```python
from build123d import *

# Parameters (mm, degrees)
SKETCH_1_R      = 2.05
EXTRUDE_1_DEPTH = 3
FILLET_1_R      = 1


with BuildPart() as part:
    # 草图1 → 凸台-拉伸1 (new body)
    with BuildSketch(Plane.XY):
        with BuildLine():
            Line((8, -14.5), (11.5, -14.5))
            Line((11.5, -14.5), (11.5, -12.41))
            ThreePointArc((11.5, -12.41), (10.495, -11.405), (11.5, -10.4))
            Line((11.5, -10.4), (14.5, -10.4))
            Line((14.5, -10.4), (14.5, -3.6))
            Line((14.5, -3.6), (11.5, -3.6))
            ThreePointArc((11.5, -3.6), (10.495, -2.595), (11.5, -1.59))
            Line((11.5, -1.59), (11.5, 1.59))
            ThreePointArc((11.5, 1.59), (10.495, 2.595), (11.5, 3.6))
            Line((11.5, 3.6), (14.5, 3.6))
            Line((14.5, 3.6), (14.5, 10.4))
            Line((14.5, 10.4), (11.5, 10.4))
            ThreePointArc((11.5, 10.4), (10.495, 11.405), (11.5, 12.41))
            Line((11.5, 12.41), (11.5, 14.5))
            Line((11.5, 14.5), (7, 14.5))
            ThreePointArc((7, 14.5), (5.95, 13.45), (4.9, 14.5))
            Line((4.9, 14.5), (4.9, 17.5))
            Line((4.9, 17.5), (-4.9, 17.5))
            Line((-4.9, 17.5), (-4.9, 14.5))
            ThreePointArc((-4.9, 14.5), (-5.95, 13.45), (-7, 14.5))
            Line((-7, 14.5), (-11.5, 14.5))
            Line((-11.5, 14.5), (-11.5, 12.41))
            ThreePointArc((-11.5, 12.41), (-10.789357685, 12.115642315), (-10.495, 11.405))
            ThreePointArc((-10.495, 11.405), (-10.789357685, 10.694357685), (-11.5, 10.4))
            Line((-11.5, 10.4), (-14.5, 10.4))
            Line((-14.5, 10.4), (-14.5, 3.6))
            Line((-14.5, 3.6), (-11.5, 3.6))
            ThreePointArc((-11.5, 3.6), (-10.789357685, 3.305642315), (-10.495, 2.595))
            ThreePointArc((-10.495, 2.595), (-10.789357685, 1.884357685), (-11.5, 1.59))
            Line((-11.5, 1.59), (-11.5, -1.59))
            ThreePointArc((-11.5, -1.59), (-10.789357685, -1.884357685), (-10.495, -2.595))
            ThreePointArc((-10.495, -2.595), (-10.789357685, -3.305642315), (-11.5, -3.6))
            Line((-11.5, -3.6), (-14.5, -3.6))
            Line((-14.5, -3.6), (-14.5, -10.4))
            Line((-14.5, -10.4), (-11.5, -10.4))
            ThreePointArc((-11.5, -10.4), (-10.789357685, -10.694357685), (-10.495, -11.405))
            ThreePointArc((-10.495, -11.405), (-10.789357685, -12.115642315), (-11.5, -12.41))
            Line((-11.5, -12.41), (-11.5, -14.5))
            Line((-11.5, -14.5), (-8, -14.5))
            ThreePointArc((-8, -14.5), (-6.95, -13.45), (-5.9, -14.5))
            Line((-5.9, -14.5), (-5.9, -17.5))
            Line((-5.9, -17.5), (5.9, -17.5))
            Line((5.9, -17.5), (5.9, -14.5))
            ThreePointArc((5.9, -14.5), (6.95, -13.45), (8, -14.5))
        make_face()
        with Locations((-7, -7)):
            Circle(SKETCH_1_R, mode=Mode.SUBTRACT)
        with Locations((7, -7)):
            Circle(SKETCH_1_R, mode=Mode.SUBTRACT)
        Polygon((-7.5, 0.890105817), (-7.5, 8.609894183), (-2.465355414, 4.75), align=None, mode=Mode.SUBTRACT)
        Polygon((5.034644586, -1), (-5.034644586, -1), (0, 2.859894183), align=None, mode=Mode.SUBTRACT)
        Polygon((-5.034644586, 10.5), (5.034644586, 10.5), (0, 6.640105817), align=None, mode=Mode.SUBTRACT)
        Polygon((2.465355414, 4.75), (7.5, 8.609894183), (7.5, 0.890105817), align=None, mode=Mode.SUBTRACT)
    extrude(amount=EXTRUDE_1_DEPTH)

    # 圆角1
    fillet_1_edges = [part.edges().sort_by_distance(p)[0] for p in [
        (5.034644586, -1, 1.5),
        (0, 2.859894183, 1.5),
        (-7.5, 8.609894183, 1.5),
        (-7.5, 0.890105817, 1.5),
        (-2.465355414, 4.75, 1.5),
        (0, 6.640105817, 1.5),
        (5.034644586, 10.5, 1.5),
        (-5.034644586, 10.5, 1.5),
        (7.5, 0.890105817, 1.5),
        (7.5, 8.609894183, 1.5),
        (2.465355414, 4.75, 1.5),
        (-5.034644586, -1, 1.5),
    ]]
    fillet(fillet_1_edges, radius=FILLET_1_R)


solid = part.part
```
Design review of the part built by this model. Coordinates are the model's own, in mm. A direction names the side the tool comes from. Give positions to 0.01 mm unless a question says otherwise; leave off trailing zeros. Write each loop counter-clockwise with the first axis right and the second up, starting at its lowest first coordinate (ties: lowest second). Pieces come first, ordered by that corner, then holes.
(1) Add section B-B (y = -5.5). Give the boundary of the cut face in (x, z), and give its area (3 significant figures).
Checked values:
outline: (-14.5, 0) - (-8.4, 0) - (-8.4, 3) - (-14.5, 3) - close; (-5.6, 0) - (5.6, 0) - (5.6, 3) - (-5.6, 3) - close; (8.4, 0) - (14.5, 0) - (14.5, 3) - (8.4, 3) - close
area: 70.2 mm2
(2) Add section A-A (x = 0). Give the boundary of the cut face in (y, z), and give its area (3 significant figures).
Checked values:
outline: (-17.5, 0) - (-1, 0) - (-1, 3) - (-17.5, 3) - close; (2.6, 0) - (6.9, 0) - (6.9, 3) - (2.6, 3) - close; (10.5, 0) - (17.5, 0) - (17.5, 3) - (10.5, 3) - close
area: 83.4 mm2
(3) Add section D-D (y = -2). Give the boundary of the cut face in (x, z), and give its area (3 significant figures).
Checked values:
outline: (-10.69, 0) - (10.69, 0) - (10.69, 3) - (-10.69, 3) - close
area: 64.1 mm2
(4) Wall thickness on line 1 along Y through (x, z) = (-2, 2.35); line 2 along Y through (x, z) = (0.5, 0.65); line 3 along X through (y, z) = (14, 2): over which ranges is each line inside the solid? List them lowest first.
Checked values:
line 1: y = -17.5 to -1, 1.33 to 8.17, 10.5 to 17.5
line 2: y = -17.5 to -1, 2.47 to 7.03, 10.5 to 17.5
line 3: x = -11.5 to -6.87, -5.03 to 5.03, 6.87 to 11.5
(5) Mouldability with a two-part tool opening along Y and no side actions: class faces 4 (the face through (6.93, -13.45, 1.48)), 5 (the face through (-11.5, 13, 1)), 6 (the face through (-1.67, 1.58, 1.48)) as +Y half, -Y half, draft (parallel to the pull), parting line (faces both ways), or undercut.
Checked values:
face 4: -Y half
face 5: draft
face 6: undercut
(6) Clearance check with flat-ended pins moving along their axes: pin 1 Ø0.9 at (x, z) = (13, 1) entering from +Y; pin 2 Ø1.7 at (y, z) = (-13, 1) entering from +X; pin 3 Ø1 at (x, y) = (6.5, -3.5) entering from -Z; pin 4 Ø0.9 at (x, z) = (-13, 1.5) entering from -Y. State where each tip first meets the part, or that it passes through.
Checked values:
pin 1: stops at y = 10.4
pin 2: stops at x = 11.5
pin 3: stops at z = 0
pin 4: stops at y = -10.4
(7) Tool access review of faces 1 (the face through (5.9, -16, 1)), 2 (the face through (13, 3.6, 1)), 3 (the face through (3.04, 9.8, 1.52)): name each direction out of +Z, -Z, +X, -X, +Y, -Y from which nothing blocks a thin tool from reaching the whole face with its end or side.
Checked values:
face 1: +Z, -Z, +X, -Y
face 2: +Z, -Z, +X
face 3: +Z, -Z
(8) Add section C-C (z = 1.25). Give the number of separate pieces and of enclosed holes in the cut face, and give its area (3 significant figures).
Checked values:
separate pieces: 1
enclosed holes: 6
area: 701 mm2
